Part model, mm, in its own coordinate system. A direction names the side the tool comes from. Round coordinates to 2 decimals unless told otherwise and drop trailing zeros. Write each loop counter-clockwise with the first axis right and the second up, starting at its lowest first coordinate (ties: lowest second). Pieces come first, ordered by that corner, then holes.
```python
from build123d import *

# Parameters (mm, degrees)
BOSS_EXTRUDE1_DEPTH         = 170
SKETCH3_W                   = 20
SKETCH3_H                   = 25
SKETCH3_W_2                 = 30
SKETCH3_H_2                 = 30
BOSS_EXTRUDE2_DEPTH         = 5
FILLET1_R                   = 5
BOSS_EXTRUDE5_DEPTH         = 15
CHAMFER1_SIZE               = 5
FILLET2_R                   = 5
SKETCH18_W                  = 20
SKETCH18_H                  = 165
CUT_EXTRUDE9_DEPTH          = 5
SKETCH21_W                  = 20
SKETCH21_H                  = 165
CUT_EXTRUDE10_DEPTH         = 5
M4_TAPPED_HOLE1_D           = 3.3
M4_TAPPED_HOLE1_DEPTH       = 5
M4_TAPPED_HOLE1_CSINK_D     = 4.05
M4_TAPPED_HOLE1_CSINK_ANGLE = 90
M4_TAPPED_HOLE1_TIP         = 0.991420021
M6_TAPPED_HOLE1_D           = 5
M6_TAPPED_HOLE1_DEPTH       = 5
M6_TAPPED_HOLE1_CSINK_D     = 6.05
M6_TAPPED_HOLE1_CSINK_ANGLE = 90
M6_TAPPED_HOLE1_TIP         = 1.502151548
M6_TAPPED_HOLE2_D           = 5
M6_TAPPED_HOLE2_DEPTH       = 5
M6_TAPPED_HOLE2_TIP         = 1.502151548
SKETCH31_R                  = 5
CUT_EXTRUDE11_DEPTH         = 267.282275039


with BuildPart() as part:
    # Sketch1 → Boss-Extrude1 (new body)
    with BuildSketch(Plane(origin=(0, 0, 0), x_dir=(1, 0, 0), z_dir=(0, 1, 0))):
        Polygon((162.5, 80), (162.5, -80), (152.5, -80), (147.5, -80), (132.5, -80), (132.5, -95), (132.5, -100), (132.5, -110), (-102.5, -110), (-102.5, -100), (-102.5, -85), (-112.5, -85), (-122.5, -85), (-122.5, -100), (-122.5, -110), (-162.5, -110), (-162.5, -100), (-162.5, -95), (-132.5, -95), (-132.5, -85), (-132.5, -75), (-93.003639463, -75), (-93.003639463, -100), (122.5, -100), (122.5, -70), (152.5, -70), (152.5, 70), (122.5, 70), (122.5, 100), (-93.003639463, 100), (-93.003639463, 75), (-132.5, 75), (-132.5, 85), (-132.5, 95), (-162.5, 95), (-162.5, 100), (-162.5, 110), (-122.5, 110), (-122.5, 100), (-122.5, 85), (-112.5, 85), (-102.5, 85), (-102.5, 100), (-102.5, 110), (132.5, 110), (132.5, 100), (132.5, 95), (132.5, 80), (147.5, 80), (152.5, 80), align=None)
    extrude(amount=BOSS_EXTRUDE1_DEPTH)

    # Sketch3 → Boss-Extrude2 (add)
    with BuildSketch(Plane(origin=(0, 0, 0), x_dir=(1, 0, 0), z_dir=(0, 1, 0))):
        with Locations((-112.5, -97.5)):
            Rectangle(SKETCH3_W, SKETCH3_H)
        Polygon((147.5, -80), (132.5, -80), (132.5, -110), (162.5, -110), (162.5, -80), align=None)
        with Locations((-112.5, 97.5)):
            Rectangle(SKETCH3_W, SKETCH3_H)
        with Locations((147.5, 95)):
            Rectangle(SKETCH3_W_2, SKETCH3_H_2)
    extrude(amount=BOSS_EXTRUDE2_DEPTH)

    # Fillet1
    fillet1_edges = [part.edges().sort_by_distance(p)[0] for p in [
        (-122.5, 87.5, 85),
        (-102.5, 87.5, 85),
        (132.5, 87.5, 80),
        (132.5, 87.5, -80),
        (-102.5, 87.5, -85),
        (-122.5, 87.5, -85),
    ]]
    fillet(fillet1_edges, radius=FILLET1_R)

    # Sketch10 → Boss-Extrude5 (add)
    with BuildSketch(Plane(origin=(0, 170, 0), x_dir=(1, 0, 0), z_dir=(0, 1, 0))):
        Polygon((-162.5, 95), (-162.5, -95), (-162.5, -100), (-162.5, -110), (-122.5, -110), (-122.5, -100), (-122.5, -85), (-112.5, -85), (-102.5, -85), (-102.5, -100), (-102.5, -110), (132.5, -110), (132.5, -100), (132.5, -95), (132.5, -80), (147.5, -80), (152.5, -80), (162.5, -80), (162.5, 80), (152.5, 80), (147.5, 80), (132.5, 80), (132.5, 95), (132.5, 100), (132.5, 110), (-102.5, 110), (-102.5, 100), (-102.5, 85), (-112.5, 85), (-122.5, 85), (-122.5, 100), (-122.5, 110), (-162.5, 110), (-162.5, 100), align=None)
    extrude(amount=BOSS_EXTRUDE5_DEPTH)

    # Chamfer1
    chamfer1_edges = [part.edges().sort_by_distance(p)[0] for p in [
        (147.5, 185, -80),
        (15, 185, -110),
        (-142.5, 185, -110),
        (-142.5, 185, 110),
        (15, 185, 110),
        (147.5, 185, 80),
    ]]
    chamfer(chamfer1_edges, length=CHAMFER1_SIZE)

    # Fillet2
    fillet2_edges = [part.edges().sort_by_distance(p)[0] for p in [
        (-122.5, 177.5, -85),
        (-102.5, 177.5, -85),
        (132.5, 175, -80),
        (132.5, 175, 80),
        (-102.5, 177.5, 85),
        (-122.5, 177.5, 85),
    ]]
    fillet(fillet2_edges, radius=FILLET2_R)

    # Sketch18 → Cut-Extrude9 (cut)
    with BuildSketch(Plane.XY.offset(110)):
        with Locations((-35, 97.5)):
            Rectangle(SKETCH18_W, SKETCH18_H)
        with Locations((-10, 97.5)):
            Rectangle(SKETCH18_W, SKETCH18_H)
        with Locations((15, 97.5)):
            Rectangle(SKETCH18_W, SKETCH18_H)
        with Locations((40, 97.5)):
            Rectangle(SKETCH18_W, SKETCH18_H)
        with Locations((65, 97.5)):
            Rectangle(SKETCH18_W, SKETCH18_H)
        with Locations((90, 97.5)):
            Rectangle(SKETCH18_W, SKETCH18_H)
        with Locations((115, 97.5)):
            Rectangle(SKETCH18_W, SKETCH18_H)
        with Locations((-85, 97.5)):
            Rectangle(SKETCH18_W, SKETCH18_H)
        with Locations((-60, 97.5)):
            Rectangle(SKETCH18_W, SKETCH18_H)
    extrude(amount=-CUT_EXTRUDE9_DEPTH, mode=Mode.SUBTRACT)

    # Sketch21 → Cut-Extrude10 (cut)
    with BuildSketch(Plane(origin=(0, 0, -110), x_dir=(-1, 0, 0), z_dir=(0, 0, -1))):
        with Locations((-90, 97.5)):
            Rectangle(SKETCH21_W, SKETCH21_H)
        with Locations((-65, 97.5)):
            Rectangle(SKETCH21_W, SKETCH21_H)
        with Locations((-40, 97.5)):
            Rectangle(SKETCH21_W, SKETCH21_H)
        with Locations((-15, 97.5)):
            Rectangle(SKETCH21_W, SKETCH21_H)
        with Locations((10, 97.5)):
            Rectangle(SKETCH21_W, SKETCH21_H)
        with Locations((35, 97.5)):
            Rectangle(SKETCH21_W, SKETCH21_H)
        with Locations((60, 97.5)):
            Rectangle(SKETCH21_W, SKETCH21_H)
        with Locations((85, 97.5)):
            Rectangle(SKETCH21_W, SKETCH21_H)
        with Locations((-115, 97.5)):
            Rectangle(SKETCH21_W, SKETCH21_H)
    extrude(amount=-CUT_EXTRUDE10_DEPTH, mode=Mode.SUBTRACT)

    # M4 Tapped Hole1
    with Locations(Plane(origin=(0, 0, 0), x_dir=(-1, 0, 0), z_dir=(0, -1, 0))):
        with Locations((-157.5, 35), (-157.5, -35), (-67.5, -105), (32.5, -105), (32.5, 105), (-67.5, 105)):
            CounterSinkHole(M4_TAPPED_HOLE1_D / 2, M4_TAPPED_HOLE1_CSINK_D / 2, depth=M4_TAPPED_HOLE1_DEPTH, counter_sink_angle=M4_TAPPED_HOLE1_CSINK_ANGLE)
            with Locations((0, 0, -(M4_TAPPED_HOLE1_DEPTH + M4_TAPPED_HOLE1_TIP / 2))):  # 118° drill point
                Cone(0, M4_TAPPED_HOLE1_D / 2, M4_TAPPED_HOLE1_TIP, mode=Mode.SUBTRACT)

    # M6 Tapped Hole1
    with Locations(Plane.ZY.offset(132.5)):
        with Locations((-85, 25), (-85, 165), (85, 165), (85, 25)):
            CounterSinkHole(M6_TAPPED_HOLE1_D / 2, M6_TAPPED_HOLE1_CSINK_D / 2, depth=M6_TAPPED_HOLE1_DEPTH, counter_sink_angle=M6_TAPPED_HOLE1_CSINK_ANGLE)
            with Locations((0, 0, -(M6_TAPPED_HOLE1_DEPTH + M6_TAPPED_HOLE1_TIP / 2))):  # 118° drill point
                Cone(0, M6_TAPPED_HOLE1_D / 2, M6_TAPPED_HOLE1_TIP, mode=Mode.SUBTRACT)

    # M6 Tapped Hole2
    with Locations(Plane.ZY.offset(162.5)):
        with Locations((-102.5, 85), (-102.5, 177.5), (0, 177.5), (102.5, 177.5), (102.5, 85)):
            Hole(M6_TAPPED_HOLE2_D / 2, depth=M6_TAPPED_HOLE2_DEPTH)
            with Locations((0, 0, -(M6_TAPPED_HOLE2_DEPTH + M6_TAPPED_HOLE2_TIP / 2))):  # 118° drill point
                Cone(0, M6_TAPPED_HOLE2_D / 2, M6_TAPPED_HOLE2_TIP, mode=Mode.SUBTRACT)

    # Sketch31 → Cut-Extrude11 (cut, through all)
    with BuildSketch(Plane(origin=(0, 5, 0), x_dir=(1, 0, 0), z_dir=(0, 1, 0))):
        with Locations(Location((147.5, 95, 0), (0, 0, 270))):
            Circle(SKETCH31_R)
        with Locations(Location((-112.5, 95, 0), (0, 0, 270))):
            Circle(SKETCH31_R)
        with Locations(Location((-112.5, -95, 0), (0, 0, 270))):
            Circle(SKETCH31_R)
        with Locations(Location((147.5, -95, 0), (0, 0, 270))):
            Circle(SKETCH31_R)
    extrude(amount=-CUT_EXTRUDE11_DEPTH, mode=Mode.SUBTRACT)


solid = part.part
```
Q1. Cut at B-B on z = 22.5. Write the cut outline in (x, y), plus the area to 4 significant figures.
Values follow:
outline: (-162.5, 170) - (152.5, 170) - (152.5, 0) - (162.5, 0) - (162.5, 185) - (-162.5, 185) - close
area: 6,575 mm2
Q2. Which spindle directions (+Z, -Z, +X, -X, +Y, -Y) get a long thin tool onto all of the face, cutting with end or side? Do faces 4 (the flat face through (65, 99, 105)), 5 (the flat face through (115, 99, -105)), 6 (the flat face through (-148, 84, 95)), 7 (the flat face through (-113, 94, 85)). Say none if no direction does.
Values follow:
face 4: +Z
face 5: -Z
face 6: -X, -Y
face 7: +Z, +Y
Q3. Wall check: L1, parallel to Z at x = 157, y = 2; L2, parallel to Z at x = 67.5, y = 3.85; L3, parallel to X at y = 2.75, z = -105. Give the ranges that are in metal, low to high.
Values follow:
L1: z = -110 to -36.57, -33.43 to 33.43, 36.57 to 110
L2: z = -110 to -106.65, -103.35 to -100, 100 to 103.35, 106.65 to 110
L3: x = -162.5 to -34.15, -30.85 to 65.85, 69.15 to 162.5
Q4. Mould opens along X. For faces 1 (the flat face through (23, 0, 105)), 2 (the flat face through (-122.5, 94, 100)), 3 (the flat face through (-132.5, 84, 85)) say: +X half, -X half, draft (parallel to the pull), parting line (faces both ways), or undercut.
Values follow:
face 1: draft
face 2: undercut
face 3: -X half
Q5. Cut at A-A on x = -112.5. Write the cut outline in (y, z), plus the area to 3 significant figures.
Values follow:
outline: (0, -110) - (5, -110) - (5, -100) - (0, -100) - close; (0, -90) - (5, -90) - (5, -85) - (185, -85) - (185, 85) - (5, 85) - (5, 90) - (0, 90) - (0, 75) - (170, 75) - (170, -75) - (0, -75) - close; (0, 100) - (5, 100) - (5, 110) - (0, 110) - close
area: 6,100 mm2
Q6. Cut at C-C on x = 94.5. Write the cut outline in (y, z), plus the area to 4 significant figures.
Values follow:
outline: (0, -110) - (15, -110) - (15, -105) - (180, -105) - (180, -110) - (185, -105) - (185, 105) - (180, 110) - (180, 105) - (15, 105) - (15, 110) - (0, 110) - (0, 100) - (170, 100) - (170, -100) - (0, -100) - close
area: 5,025 mm2
Q7. Drop flat-ended pins along their axis: pin 1 (16 mm diameter, centred on x = -112.5, z = 95, fed in from +Y); pin 2 (16 mm diameter, centred on x = 90, y = 99.5, fed in from +Z); pin 3 (5.5 mm diameter, centred on y = 60, z = -107.5, fed in from +X). Give the stop position or say it passes through.
Values follow:
pin 1: stops at y = 5
pin 2: stops at z = 105
pin 3: stops at x = 132.5
Q8. Cut at D-D on x = 147.5. Write the cut outline in (y, z), plus the area to 4 significant figures.
Values follow:
outline: (0, -110) - (5, -110) - (5, -100) - (0, -100) - close; (0, -90) - (5, -90) - (5, -80) - (180, -80) - (185, -75) - (185, 75) - (180, 80) - (5, 80) - (5, 90) - (0, 90) - (0, 70) - (170, 70) - (170, -70) - (0, -70) - close; (0, 100) - (5, 100) - (5, 110) - (0, 110) - close
area: 5,975 mm2
